```python
from build123d import *

# Parameters (mm, degrees)
F0_W          = 69.85
F0_H          = 69.85
F1_DEPTH      = 3.175
F2_R          = 3.175
F3_R          = 2.2499955
F4_DEPTH      = 25.4
F4_DEPTH_BACK = 101
F6_DEPTH      = 25.4
F7_R          = 1.999996
F8_DEPTH      = 6.35
F9_R          = 6.35
F10_DEPTH     = 3.175
F11_DEPTH     = 7.62


# Not quite as in the source:
# - an extrude ends at something that could not be found from the text; its depth is read off the source's solid


with BuildPart() as f1:
    # F0 (on Top) → F1 (new body)
    with BuildSketch(Plane.XY):
        Rectangle(F0_W, F0_H)
    extrude(amount=F1_DEPTH)

    # F2
    f2_edges = [f1.edges().sort_by_distance(p)[0] for p in [
        (-34.925, -34.925, 1.5875),
        (34.925, -34.925, 1.5875),
        (34.925, 34.925, 1.5875),
        (-34.925, 34.925, 1.5875),
    ]]
    fillet(f2_edges, radius=F2_R)

    # F3 (on face) → F4 (cut, two sides)
    with BuildSketch(Plane.XY.offset(3.175)) as f4_sk:
        with Locations((-31.75, 31.75)):
            Circle(F3_R)
        with Locations((31.75, 31.75)):
            Circle(F3_R)
        with Locations((31.75, -31.75)):
            Circle(F3_R)
        with Locations((-31.75, -31.75)):
            Circle(F3_R)
    extrude(amount=-F4_DEPTH, mode=Mode.SUBTRACT)
    extrude(f4_sk.sketch, amount=F4_DEPTH_BACK, mode=Mode.SUBTRACT)

    # F5 (on face) → F6 (join)
    with BuildSketch(Plane.XY.offset(3.175)):
        with BuildLine():
            Line((25.4, 34.925), (-25.4, 34.925))
            ThreePointArc((-25.4, 34.925), (-27.6450640303, 33.9950640303), (-28.575, 31.75))
            Line((-28.575, 31.75), (-28.575, -31.75))
            ThreePointArc((-28.575, -31.75), (-27.6450640303, -33.9950640303), (-25.4, -34.925))
            Line((-25.4, -34.925), (25.4, -34.925))
            ThreePointArc((25.4, -34.925), (27.6450640303, -33.9950640303), (28.575, -31.75))
            Line((28.575, -31.75), (28.575, 31.75))
            ThreePointArc((28.575, 31.75), (27.6450640303, 33.9950640303), (25.4, 34.925))
        make_face()
        with BuildLine():
            ThreePointArc((-25.4, 28.575), (-23.1549359697, 29.5049359697), (-22.225, 31.75))
            Line((-22.225, 31.75), (22.225, 31.75))
            ThreePointArc((22.225, 31.75), (23.1549359697, 29.5049359697), (25.4, 28.575))
            Line((25.4, 28.575), (25.4, -28.575))
            ThreePointArc((25.4, -28.575), (23.1549359697, -29.5049359697), (22.225, -31.75))
            Line((22.225, -31.75), (-22.225, -31.75))
            ThreePointArc((-22.225, -31.75), (-23.1549359697, -29.5049359697), (-25.4, -28.575))
            Line((-25.4, -28.575), (-25.4, 28.575))
        make_face(mode=Mode.SUBTRACT)
    extrude(amount=F6_DEPTH)

    # F7 (on face) → F8 (cut)
    with BuildSketch(Plane.XY.offset(28.575)):
        with Locations((-25.4, 31.75)):
            Circle(F7_R)
        with Locations((25.4, 31.75)):
            Circle(F7_R)
        with Locations((25.4, -31.75)):
            Circle(F7_R)
        with Locations((-25.4, -31.75)):
            Circle(F7_R)
    extrude(amount=-F8_DEPTH, mode=Mode.SUBTRACT)

    # F9 (on face) → F10 (cut, through all)
    with BuildSketch(Plane.XZ.offset(34.925)):
        with Locations((-14.2875, 15.875)):
            Circle(F9_R)
    extrude(amount=-F10_DEPTH, mode=Mode.SUBTRACT)

    # F11 (add): a face of the model
    f11_faces = [f1.faces().sort_by_distance(p)[0] for p in [
        (0, 34.0224954294, 28.575),
    ]]
    extrude(f11_faces, amount=F11_DEPTH)


solid = f1.part
```
CAD build for the part. Positions are in the model's coordinates, mm. A direction names the side the tool comes from. Give positions to 0.01 mm unless a question says otherwise; leave off trailing zeros. Loops run counter-clockwise (first coordinate to the right, second up) from the corner with the lowest first, then second, coordinate; pieces in that order, holes last. Notation, with made-up numbers: (-16.75, 10.25) -> (28.25, 10.25) arc R5 cw to (28.25, 18.25) -> close; hole circle Ø11 at (-31, -24.75). An arc over 180 degrees is marked (long way). Use a Markdown table: item, result.
1. Flat gauge pins, fed straight in: pin 1 (5 mm diameter, centred on x = -31.75, y = -31.75, fed in from +Z) (3 decimals); pin 2 (5 mm diameter, centred on y = 25, z = 29.5, fed in from +X) (3 decimals); pin 3 (3.5 mm diameter, centred on x = -25.4, y = 31.75, fed in from +Z) (3 decimals). Where does each tip first touch, or does it go through?
Check result:
| item | result |
|---|---|
| pin 1 | stops at z = 3.175 |
| pin 2 | stops at x = 28.575 |
| pin 3 | stops at z = 22.225 |
2. Wall check: L1, parallel to X at y = 0, z = 6 (3 decimals); L2, parallel to Y at x = -17, z = 27.5 (3 decimals). Give the ranges that are in metal, low to high. Write a range as [from, to].
Check result:
| item | result |
|---|---|
| L1 | x = [-28.575, -25.4], [25.4, 28.575] |
| L2 | y = [-34.925, -31.75], [31.75, 34.925] |
3. Slice it at C-C (x = 11.5). List the corners of the cut face in (y, z) (3 decimals), plus the area to 3 significant figures.
Check result:
| item | result |
|---|---|
| outline | (-34.925, 0) -> (34.925, 0) -> (34.925, 36.195) -> (31.75, 36.195) -> (31.75, 3.175) -> (-31.75, 3.175) -> (-31.75, 36.195) -> (-34.925, 36.195) -> close |
| area | 431 mm^2 |
4. Which spindle directions (+Z, -Z, +X, -X, +Y, -Y) get a long thin tool onto all of the face, cutting with end or side? Do faces 1 (the cylindrical face through (27.67, 33.97, 19.45)), 2 (the flat face through (28.575, 0, 19)), 3 (the flat face through (0, -31.75, 19)). Say none if no direction does.
Check result:
| item | result |
|---|---|
| face 1 | +Z, +X, +Y |
| face 2 | +Z, +X, +Y, -Y |
| face 3 | +Z |
5. Slice it at B-B (y = 23.5). List the corners of the cut face in (x, z) (3 decimals).
Check result:
| item | result |
|---|---|
| outline | (-34.925, 0) -> (34.925, 0) -> (34.925, 3.175) -> (28.575, 3.175) -> (28.575, 36.195) -> (25.4, 36.195) -> (25.4, 3.175) -> (-25.4, 3.175) -> (-25.4, 36.195) -> (-28.575, 36.195) -> (-28.575, 3.175) -> (-34.925, 3.175) -> close |
6. Mould opens along X. For faces 4 (the flat face through (-34.925, 0, 2)), 5 (the flat face through (-25, -32, 22.225)), 6 (the flat face through (34.925, 0, 2)) say: pulls with the +X half, pulls with the -X half, needs draft (parallel to the pull), parting line crosses it, or undercut.
Check result:
| item | result |
|---|---|
| face 4 | pulls with the -X half |
| face 5 | undercut |
| face 6 | pulls with the +X half |
7. Slice it at A-A (z = 31.5). List the corners of the cut face in (x, y) (3 decimals).
Check result:
| item | result |
|---|---|
| outline | (-28.575, -31.75) arc R3.175 ccw to (-25.4, -34.925) -> (25.4, -34.925) arc R3.175 ccw to (28.575, -31.75) -> (28.575, 31.75) arc R3.175 ccw to (25.4, 34.925) -> (-25.4, 34.925) arc R3.175 ccw to (-28.575, 31.75) -> close; hole circle Ø4 at (-25.4, -31.75); hole circle Ø4 at (-25.4, 31.75); hole (-25.4, -28.575) arc R3.175 cw to (-22.225, -31.75) -> (22.225, -31.75) arc R3.175 cw to (25.4, -28.575) -> (25.4, 28.575) arc R3.175 cw to (22.225, 31.75) -> (-22.225, 31.75) arc R3.175 cw to (-25.4, 28.575) -> close; hole circle Ø4 at (25.4, -31.75); hole circle Ø4 at (25.4, 31.75) |
8. Slice it at D-D (z = 8). List the corners of the cut face in (x, y) (3 decimals), plus the area to 3 significant figures.
Check result:
| item | result |
|---|---|
| outline | (-28.575, -31.75) arc R3.175 ccw to (-25.4, -34.925) -> (25.4, -34.925) arc R3.175 ccw to (28.575, -31.75) -> (28.575, 31.75) arc R3.175 ccw to (25.4, 34.925) -> (-25.4, 34.925) arc R3.175 ccw to (-28.575, 31.75) -> close; hole (-25.4, -28.575) arc R3.175 cw to (-22.225, -31.75) -> (22.225, -31.75) arc R3.175 cw to (25.4, -28.575) -> (25.4, 28.575) arc R3.175 cw to (22.225, 31.75) -> (-22.225, 31.75) arc R3.175 cw to (-25.4, 28.575) -> close |
| area | 789 mm^2 |
